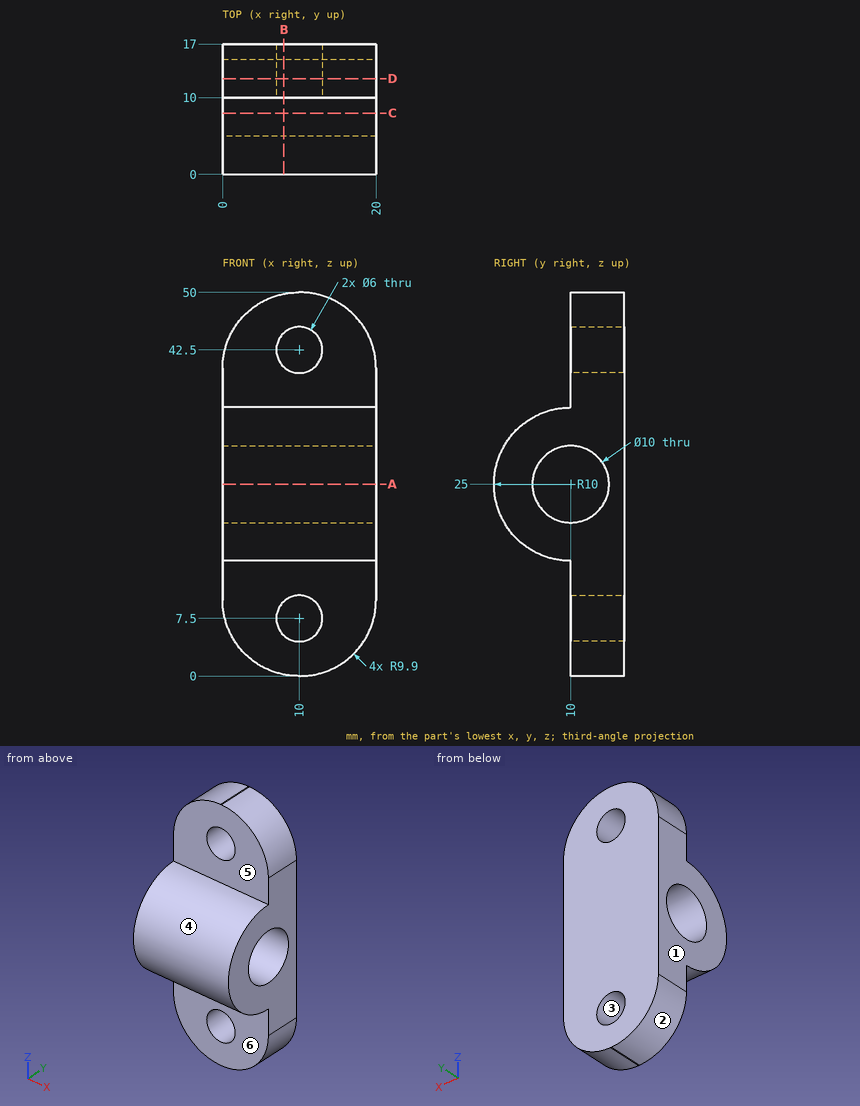
Job drawing, mm, ordinate dimensions from the low corner. One solid piece. A direction names the side the tool comes from. Coordinates: 2 decimals unless noted, no trailing zeros. Loops run counter-clockwise (first coordinate to the right, second up) from the corner with the lowest first, then second, coordinate; pieces in that order, holes last. Notation, with made-up numbers: (-10, 26) -> (5, 26) arc R8 ccw to (5, 37) -> close; hole circle Ø5 at (27.5, 77). An arc over 180 degrees is marked (long way). One line per item, written item: value.
1. Flat gauge pins, fed straight in: P1, Ø7.5, axis at x = 8.5, z = 44, coming from the -Y side; P2, Ø8, axis at x = 14.5, y = 10.5, coming from the +Z side; P3, Ø4, axis at x = 6.5, y = 4, coming from the +Z side. Where does each tip first touch, or does it go through?
Answers:
P1: stops at y = 10
P2: stops at z = 49.99
P3: stops at z = 34.17
2. Which spindle directions (+Z, -Z, +X, -X, +Y, -Y) get a long thin tool onto all of the face, cutting with end or side? Do the marked faces 4, 5 and 6. Say none if no direction does.
Answers:
face 4: +X, -X, -Y
face 5: +Z, +X, -X, -Y
face 6: -Z, +X, -X, -Y
3. Pull direction Z, two halves, no side cores. Call the marked faces 1, 2 and 3: pulls with the +Z half, pulls with the -Z half, needs draft (parallel to the pull), parting line crosses it, or undercut.
Answers:
face 1: needs draft
face 2: pulls with the -Z half
face 3: undercut
4. Slice it at C-C on y = 8. Write the cut outline in (x, z).
Answers:
outline: (0, 15.2) -> (20, 15.2) -> (20, 20.42) -> (0, 20.42) -> close; (0, 29.58) -> (20, 29.58) -> (20, 34.8) -> (0, 34.8) -> close
5. Drill centre lines: line 1 (Z direction, x = 10, y = 15.5); line 2 (Y direction, x = 11, z = 25); line 3 (Z direction, x = 10, y = 12.25). Where is each one in solid material? Low to high. Write a range as [from, to].
Answers:
line 1: z = [0, 4.5], [10.5, 39.5], [45.5, 50]
line 2: y = [0, 5], [15, 17]
line 3: z = [0, 4.5], [10.5, 20.53], [29.47, 39.5], [45.5, 50]
6. Slice it at A-A on z = 25. Write the cut outline in (x, y).
Answers:
outline: (0, 0) -> (20, 0) -> (20, 5) -> (0, 5) -> close; (0, 15) -> (20, 15) -> (20, 17) -> (0, 17) -> close
7. Slice it at B-B on x = 8. Write the cut outline in (y, z).
Answers:
outline: (10, 0.18) -> (17, 0.18) -> (17, 5.26) -> (10, 5.26) -> close; (10, 9.74) -> (17, 9.74) -> (17, 40.26) -> (10, 40.26) -> (10, 35) arc R10 ccw to (10, 15) -> close; (10, 44.74) -> (17, 44.74) -> (17, 49.82) -> (10, 49.82) -> close; hole circle Ø10 at (10, 25)
8. Slice it at D-D on y = 12.5. Write the cut outline in (x, z).
Answers:
outline: (0, 9.9) arc R9.9 ccw to (9.9, 0) -> (10.1, 0) arc R9.9 ccw to (20, 9.9) -> (20, 20.67) -> (0, 20.67) -> close; (0, 29.33) -> (20, 29.33) -> (20, 40.1) arc R9.9 ccw to (10.1, 50) -> (9.9, 50) arc R9.9 ccw to (0, 40.1) -> close; hole circle Ø6 at (10, 7.5); hole circle Ø6 at (10, 42.5)
